```python
from build123d import *


with BuildPart() as part:
    # Sketch1 → Revolve3 (revolve)
    with BuildSketch(Plane(origin=(0, 0, 0), x_dir=(0, 0, -1), z_dir=(1, 0, 0))):
        with BuildLine():
            Line((8.255, 9.855919884), (8.001, 9.601919884))
            Line((8.001, 9.601919884), (3.3175, 9.601919884))
            ThreePointArc((3.3175, 9.601919884), (3.092993597, 9.508926287), (3, 9.284419884))
            Line((3, 9.284419884), (3, 3.324235778))
            ThreePointArc((3, 3.324235778), (3.057419226, 3.142125259), (3.208908604, 3.025883371))
            Line((3.208908604, 3.025883371), (5.441838421, 2.213163382))
            Line((5.441838421, 2.213163382), (5.6275, 1.891588094))
            Line((5.6275, 1.891588094), (5.6275, 0.254))
            Line((5.6275, 0.254), (5.3735, 0))
            Line((5.3735, 0), (0, 0))
            Line((0, 0), (0, 12.009719884))
            Line((0, 12.009719884), (8.255, 12.009719884))
            Line((8.255, 12.009719884), (8.255, 9.855919884))
        make_face()
    revolve(axis=Axis((0, 6.004859942, -83.82), (0, 1, 0)))


solid = part.part
```
Geometry check sheet. Reference: the model listing, model coordinates, mm. A direction names the side the tool comes from. Coordinates: 2 decimals unless noted, no trailing zeros. Order: outer loops, then holes, each group sorted by start corner. A loop starts at its lowest first (then second) coordinate and runs counter-clockwise, first axis right, second up. Notation, with made-up numbers: (23, 44.25) - (81, 44.25) arc R10 cw to (81, 54.25) - close; hole circle Ø4 at (5.25, -20.75). An arc over 180 degrees is marked (long way). Answer as a JSON object with one key per item and string values. Group by question number.
Item 1: Draft check along X on faces 4 (the face through (3.69, 6.09, -167.56)), 5 (the face through (-62, 0, -133)), 6 (the face through (-29, 9.602, -155)). Enter one of: +X half, -X half, draft (parallel to the pull), parting line (faces both ways), or undercut.
Item 2: Sectioned sample at C-C, the plane y = 6.5. Record the cut outline in (x, z).
Item 3: Depth check by flat-ended pin: pin 1 Ø1.5 at (y, z) = (7.5, -72.5) entering from +X; pin 2 Ø3 at (x, y) = (52, 5.5) entering from +Z; pin 3 Ø1 at (x, y) = (43.5, 10.5) entering from +Z. Enter the tip coordinate at first touch or a pass-through.
Item 4: Tool access check on faces 1 (the face through (3.438, 1.061, -161.937)), 2 (the face through (3.322, 10.918, -159.312)), 3 (the face through (24.276, 6.263, -6.732)). Record the directions out of +Z, -Z, +X, -X, +Y, -Y that give a thin tool (end or side, any length) a straight path to the whole face; none if there is none.
Item 5: Scan lines: probe 1 along X at (y, z) = (7.5, -83.82); probe 2 along X at (y, z) = (11.5, -83.82) (3 decimals); probe 3 along Z at (x, y) = (48, 4). Record each from-to range of solid material in increasing order.
Resolved:
{
 "1": {"face 4": "parting line", "face 5": "draft", "face 6": "undercut"},
 "2": {"outline": "circle Ø167.64 at (0, -83.82); hole circle Ø161.64 at (0, -83.82)"},
 "3": {"pin 1": "x = 83.15", "pin 2": "z = -16.92", "pin 3": "z = -11.87"},
 "4": {"face 1": "-Y", "face 2": "+Y, -Y", "face 3": "none"},
 "5": {"probe 1": "-83.82 to -80.82, 80.82 to 83.82", "probe 2": "-83.82 to -75.565, 75.565 to 83.82", "probe 3": "-152.54 to -148.84, -18.8 to -15.1"}
}
